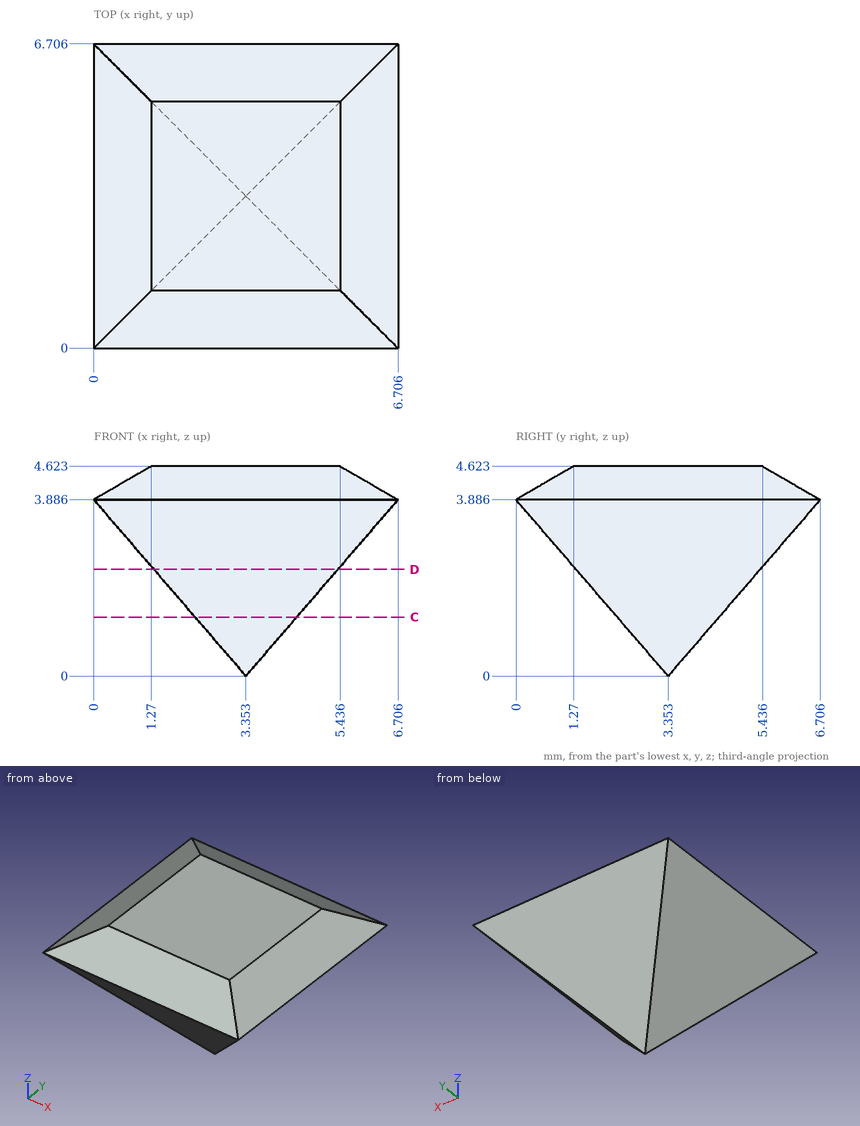
Geometry: see drawing. Coordinates: mm, zero at the bounding-box minimum. Coordinates: 2 decimals unless noted, no trailing zeros. Order: outer loops, then holes, each group sorted by start corner. A loop starts at its lowest first (then second) coordinate and runs counter-clockwise, first axis right, second up. Notation, with made-up numbers: M -36,5 L 0,5 A15 cw 0,9 Z; hole C 83,56.25 d9. An arc over 180 degrees is marked long. Answer in a Markdown table with one row per item. Add a question column.
Q1. Section query C-C on z = 1.3. Return the cut outline in (x, y) (1 decimal).
Q2. Section query D-D on z = 2.35. Return the cut outline in (x, y) (1 decimal).
Q3. Contact query for flat-ended pins moving along their axis: P1, Ø3, axis at x = 1, y = 3, coming from the -Z side; P2, Ø2, axis at x = 6, z = 2, coming from the -Y side (1 decimal); P3, Ø1.5, axis at y = 4, z = 1.5, coming from the -X side. Output: stop coordinate, or through.
Q4. Line query: L1, parallel to X at y = 3.25, z = 1.3 (1 decimal); L2, parallel to Z at x = 4.5, y = 4 (1 decimal); L3, parallel to Y at x = 1, z = 3.3 (1 decimal). Output: solid intervals per line, ascending.
Completed:
| question | item | result |
|---|---|---|
| 1 | outline | M 2.2,2.2 L 4.5,2.2 L 4.5,4.5 L 2.2,4.5 Z |
| 2 | outline | M 1.3,1.3 L 5.4,1.3 L 5.4,5.4 L 1.3,5.4 Z |
| 3 | P1 | stops at z = 0.99 |
| 3 | P2 | stops at y = 0.8 |
| 3 | P3 | stops at x = 1.41 |
| 4 | L1 | x = 2.2 to 4.5 |
| 4 | L2 | z = 1.3 to 4.6 |
| 4 | L3 | y = 0.5 to 6.2 |
